Could you check a few things on this drawing? It's one solid part, dimensions in mm from its lowest x, y, z. A direction names the side the tool comes from. Give positions to 0.01 mm unless a question says otherwise; leave off trailing zeros. Loops run counter-clockwise (first coordinate to the right, second up) from the corner with the lowest first, then second, coordinate; pieces in that order, holes last.
1. I need wall thicknesses on line 1 along X through (y, z) = (14.75, 11); line 2 along X through (y, z) = (4.75, 2.25); line 3 along Z through (x, y) = (10.5, 8.25). Which ranges of each line are inside material? Lowest first, please.
2. Imagine slicing it at D-D (z = 9.75). List the corners of the cut face in (x, y) for me.
3. For P1, Ø1.6, axis at x = 11, y = 19, coming from the -Z side; P2, Ø5, axis at x = 8, z = 12, coming from the +Y side; P3, Ø12, axis at x = 15.5, y = 17.5, coming from the -Z side, each with a flat end and sliding along its axis, tell me the tip position at first contact or that it passes through.
4. For the marked faces 1, 2, 3, 4 and 5, which set-ups out of +Z, -Z, +X, -X, +Y, -Y let a thin tool reach every point of the face, with its end or its side?
5. Imagine slicing it at C-C (x = 15.5). List the corners of the cut face in (y, z) for me.
6. Imagine slicing it at B-B (y = 3.5). List the corners of the cut face in (x, z) for me.
7. Imagine slicing it at A-A (z = 17.5). Count the separate pieces of the cut face and the enclosed holes in it.
8. Thinking about a two-plate mould opening in X: for the marked faces 6, 7, 8 and 9, which applies, +X half, -X half, draft (parallel to the pull), parting line (faces both ways), or undercut?
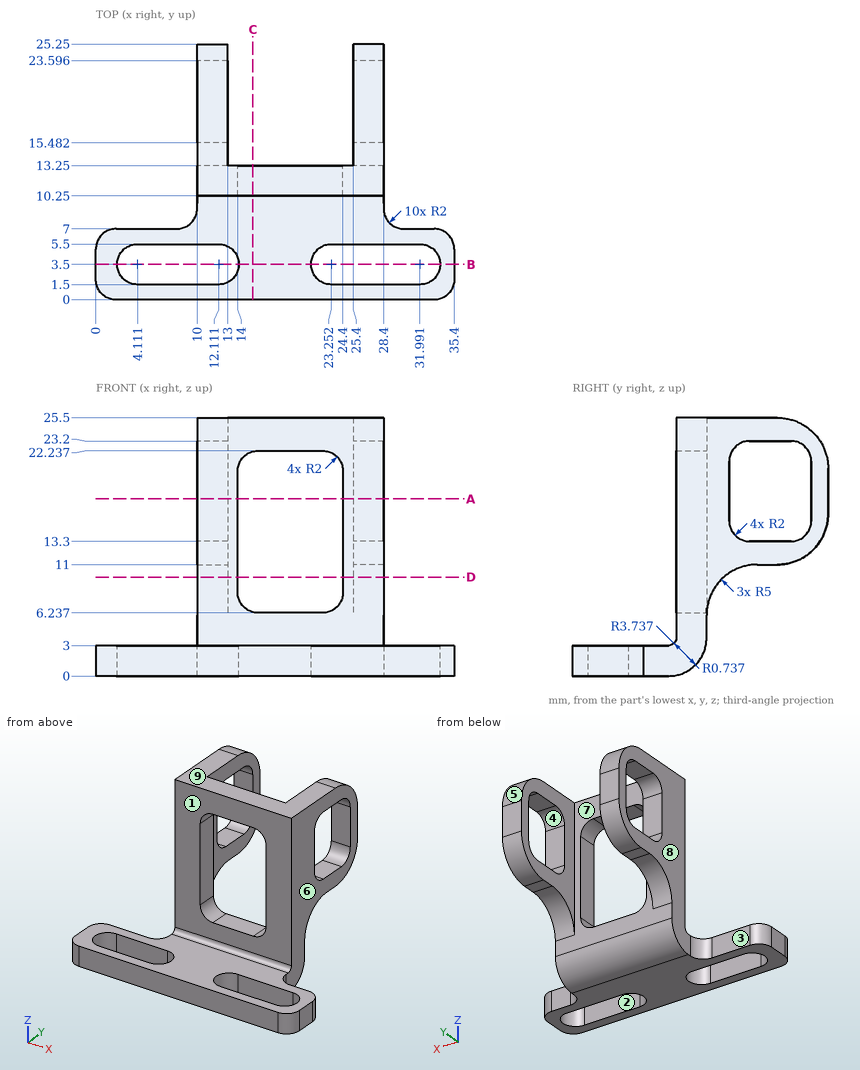
Derived:
1. line 1: x = 10 to 13, 25.4 to 28.4
1. line 2: x = 0 to 2.55, 13.67 to 21.69, 33.55 to 35.4
1. line 3: z = 0 to 3
2. outline: (10, 10.25) - (14, 10.25) - (14, 13.25) - (13, 13.25) - (13, 14.94) - (10, 14.94) - close; (24.4, 10.25) - (28.4, 10.25) - (28.4, 14.94) - (25.4, 14.94) - (25.4, 13.25) - (24.4, 13.25) - close
3. P1: stops at z = 11
3. P2: stops at y = 24.58
3. P3: stops at z = 0.57
4. face 1: +Z, +X, -X, -Y
4. face 2: +Z, -Z
4. face 3: +Z, -Z, -X, +Y
4. face 4: +X, -X
4. face 5: +Z, +X, -X, +Y
5. outline: (0, 0) - (9.51, 0) arc R3.74 ccw to (13.25, 3.74) - (13.25, 6.3) - (10.25, 6.3) - (10.25, 3.74) arc R0.74 cw to (9.51, 3) - (0, 3) - close; (10.25, 22.17) - (13.25, 22.17) - (13.25, 25.5) - (10.25, 25.5) - close
6. outline: (0, 0) - (2.11, 0) - (2.11, 3) - (0, 3) - close; (14.11, 0) - (21.25, 0) - (21.25, 3) - (14.11, 3) - close; (33.99, 0) - (35.4, 0) - (35.4, 3) - (33.99, 3) - close
7. separate pieces: 4
7. enclosed holes: 0
8. face 6: +X half
8. face 7: undercut
8. face 8: -X half
8. face 9: draft
